Here's how the part is built. I have some questions about the finished solid (model axes, mm). Face numbers are marked on the shaded views. A direction names the side the tool comes from. Coordinates: 2 decimals unless noted, no trailing zeros. Order: outer loops, then holes, each group sorted by start corner. A loop starts at its lowest first (then second) coordinate and runs counter-clockwise, first axis right, second up. Notation, with made-up numbers: (-18.5, 27) - (24.5, 27) arc R9 cw to (24.5, 33) - close; hole circle Ø11 at (40, 31.5). An arc over 180 degrees is marked (long way). Use CSV: the item, a comma, the result in double quotes. Start each with the question number.
from build123d import *

# Parameters (mm, degrees)
F0_R     = 3.5
F1_DEPTH = 2
F2_W     = 23
F2_H     = 2
F3_DEPTH = 15
F4_START = 13
F4_DEPTH = 2
F5_START = -13
F5_DEPTH = 2
F6_SIZE  = 1
F7_SIZE2 = 0.99999
F7_SIZE  = 1.99999


# Not quite as in the source:
# - a fillet or chamfer is up to 0.001 mm smaller than in the source, because OpenCascade refuses the exact size


with BuildPart() as f1:
    # F0 (on Front) → F1 (new body)
    with BuildSketch(Plane.XZ):
        Polygon((-3, 12.5), (-15, 12.5), (-15, -12.5), (15, -12.5), (15, 12.5), (3, 12.5), (3, 9.5), (-3, 9.5), align=None)
        with BuildLine():
            ThreePointArc((-6.3639610307, -8.4852813742), (-8.4852813742, -8.4852813742), (-8.4852813742, -6.3639610307))
            Line((-8.4852813742, -6.3639610307), (-6.3639610307, -4.2426406871))
            ThreePointArc((-6.3639610307, -4.2426406871), (-4.7292757104, -3.9174815601), (-3.8033008589, -5.3033008589))
            ThreePointArc((-3.8033008589, -5.3033008589), (-3.9174815601, -5.8773260074), (-4.2426406871, -6.3639610307))
            Line((-4.2426406871, -6.3639610307), (-6.3639610307, -8.4852813742))
        make_face(mode=Mode.SUBTRACT)
        with BuildLine():
            ThreePointArc((8.4852813742, -6.3639610307), (8.8104405012, -6.8505960539), (8.9246212025, -7.4246212025))
            ThreePointArc((8.9246212025, -7.4246212025), (7.998646351, -8.8104405012), (6.3639610307, -8.4852813742))
            Line((6.3639610307, -8.4852813742), (4.2426406871, -6.3639610307))
            ThreePointArc((4.2426406871, -6.3639610307), (4.2426406871, -4.2426406871), (6.3639610307, -4.2426406871))
            Line((6.3639610307, -4.2426406871), (8.4852813742, -6.3639610307))
        make_face(mode=Mode.SUBTRACT)
        with BuildLine():
            ThreePointArc((-8.4852813742, 6.3639610307), (-8.4852813742, 8.4852813742), (-6.3639610307, 8.4852813742))
            Line((-6.3639610307, 8.4852813742), (-4.2426406871, 6.3639610307))
            ThreePointArc((-4.2426406871, 6.3639610307), (-3.9174815601, 5.8773260074), (-3.8033008589, 5.3033008589))
            ThreePointArc((-3.8033008589, 5.3033008589), (-4.7292757104, 3.9174815601), (-6.3639610307, 4.2426406871))
            Line((-6.3639610307, 4.2426406871), (-8.4852813742, 6.3639610307))
        make_face(mode=Mode.SUBTRACT)
        Circle(F0_R, mode=Mode.SUBTRACT)
        with BuildLine():
            ThreePointArc((6.3639610307, 8.4852813742), (7.998646351, 8.8104405012), (8.9246212025, 7.4246212025))
            ThreePointArc((8.9246212025, 7.4246212025), (8.8104405012, 6.8505960539), (8.4852813742, 6.3639610307))
            Line((8.4852813742, 6.3639610307), (6.3639610307, 4.2426406871))
            ThreePointArc((6.3639610307, 4.2426406871), (4.2426406871, 4.2426406871), (4.2426406871, 6.3639610307))
            Line((4.2426406871, 6.3639610307), (6.3639610307, 8.4852813742))
        make_face(mode=Mode.SUBTRACT)
    extrude(amount=F1_DEPTH)

    # F2 (on Right) → F3 (join, symmetric)
    with BuildSketch(Plane.YZ):
        with Locations((11.5, -11.5)):
            Rectangle(F2_W, F2_H)
    extrude(amount=F3_DEPTH, both=True)

    # F2 (on Right) → F4 (join)
    with BuildSketch(Plane.YZ.offset(F4_START)):
        Polygon((0, 12.5), (0, -10.5), (23, -10.5), align=None)
    extrude(amount=F4_DEPTH)

    # F2 (on Right) → F5 (join)
    with BuildSketch(Plane.YZ.offset(F5_START)):
        Polygon((0, 12.5), (0, -10.5), (23, -10.5), align=None)
    extrude(amount=-F5_DEPTH)

    # F6
    f6_edges = [f1.edges().sort_by_distance(p)[0] for p in [
        (5.303301, 0, 7.424621),
        (-5.303301, 0, 7.424621),
        (-7.424621, 0, -5.303301),
        (7.424621, 0, -5.303301),
    ]]
    chamfer(f6_edges, length=F6_SIZE)

    # F7 (size 2 and 1 in the source; OpenCascade refuses exactly that, so slightly less here)
    f7_edges = [f1.edges().sort_by_distance(p)[0] for p in [
        (-3.5, -2, 0),
    ]]
    f7_side = f1.faces().sort_by_distance((-3.5, -1, 0))[0]
    chamfer(f7_edges, length=F7_SIZE, length2=F7_SIZE2, reference=f7_side)


solid = f1.part
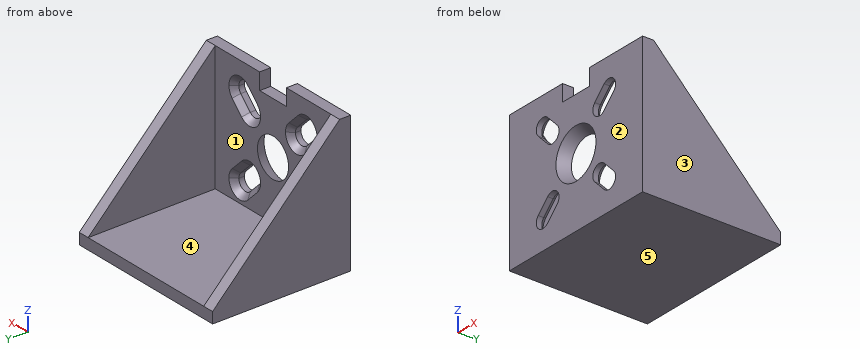
Item 1: Suppose I cut it at D-D on y = 21.5. Write out the boundary of the cut face in (x, z), then the cut area to 3 significant figures.
Item 2: Please list where these lines run through material, in increasing order: line 1 along X through (y, z) = (6.5, -2.5); line 2 along Z through (x, y) = (-5.75, -0.5); line 3 along Z through (x, y) = (3.5, 9.25). Write a range as from..to.
Item 3: Suppose I cut it at C-C on y = 4. Write out the boundary of the cut face in (x, z).
Item 4: For the marked faces 1 and 2, which set-ups out of +Z, -Z, +X, -X, +Y, -Y let a thin tool reach every point of the face, with its end or its side?
Item 5: We'd pull the mould along X, two halves only. Please class the marked faces 3, 4 and 5: released by +X, released by -X, zero draft, split by the parting line, or undercut.
Item 6: For pin 1 Ø11.5 at (x, z) = (-2, -3.5) entering from +Y; pin 2 Ø2 at (x, y) = (9, 18.5) entering from +Z, each with a flat end and sliding along its axis, tell me the tip position at first contact or that it passes through.
Here are the results:
1,outline,"(-15, -12.5) - (15, -12.5) - (15, -9) - (13, -9) - (13, -10.5) - (-13, -10.5) - (-13, -9) - (-15, -9) - close"
1,area,"66.0 mm^2"
2,line 1,"-15..-13, 13..15"
2,line 2,"-12.5..-8.58, -3.35..3.35, 8.58..12.5"
2,line 3,"-12.5..-10.5"
3,outline,"(-15, -12.5) - (15, -12.5) - (15, 8.5) - (13, 8.5) - (13, -10.5) - (-13, -10.5) - (-13, 8.5) - (-15, 8.5) - close"
4,face 1,"+Z, +Y"
4,face 2,"+Z, -Z, +X, -X, -Y"
5,face 3,"released by +X"
5,face 4,"undercut"
5,face 5,"zero draft"
6,pin 1,"y = 0"
6,pin 2,"z = -10.5"
